```python
from build123d import *

# Parameters (mm, degrees)
SKETCH2_R           = 19.05
BOSS_EXTRUDE1_DEPTH = 62.484
SKETCH3_R           = 34.671
BOSS_EXTRUDE2_DEPTH = 12.7
SKETCH4_R           = 15.621
BOSS_EXTRUDE3_DEPTH = 19.05
SKETCH5_R           = 16.891
BOSS_EXTRUDE4_DEPTH = 2.54


with BuildPart() as part:
    # Sketch1 → Revolve1 (revolve)
    with BuildSketch(Plane.XY, mode=Mode.PRIVATE) as revolve1_sk:
        Polygon((0, 0), (0, 6.985), (16.761748485, 16.6624), (188.722, 16.6624), (188.722, 34.671), (201.422, 34.671), (201.422, 19.05), (300.99, 19.05), (300.99, 34.671), (326.39, 34.671), (332.329202219, 38.1), (484.729202219, 38.1), (484.729202219, 0), align=None)
    revolve(revolve1_sk.sketch.rotate(Axis((0, 0, 0), (1, 0, 0)), 90), axis=Axis((0, 0, 0), (1, 0, 0)))  # turned: the seam where the file's is

    # Sketch2 → Boss-Extrude1 (add)
    with BuildSketch(Plane(origin=(0, 0, 0), x_dir=(1, 0, 0), z_dir=(0, 1, 0))):
        with Locations(Location((251.206, 0, 0), (0, 0, 270))):  # turned: the seam where the file's is
            Circle(SKETCH2_R)
    extrude(amount=BOSS_EXTRUDE1_DEPTH)

    # Sketch3 → Boss-Extrude2 (add)
    with BuildSketch(Plane(origin=(0, 62.484, 0), x_dir=(1, 0, 0), z_dir=(0, 1, 0))):
        with Locations(Location((251.206, 0, 0), (0, 0, 270))):  # turned: the seam where the file's is
            Circle(SKETCH3_R)
    extrude(amount=-BOSS_EXTRUDE2_DEPTH)

    # Sketch4 → Boss-Extrude3 (add)
    with BuildSketch(Plane(origin=(484.729202219, 0, 0), x_dir=(0, 0, -1), z_dir=(1, 0, 0))):
        with Locations(Location((17.272, 0, 0), (0, 0, 180))):  # turned: the seam where the file's is
            Circle(SKETCH4_R)
    extrude(amount=BOSS_EXTRUDE3_DEPTH)

    # Sketch5 → Boss-Extrude4 (add)
    with BuildSketch(Plane(origin=(484.729202219, 0, 0), x_dir=(0, 0, -1), z_dir=(1, 0, 0))):
        with Locations(Location((-19.812, 0, 0), (0, 0, 180))):  # turned: the seam where the file's is
            Circle(SKETCH5_R)
    extrude(amount=BOSS_EXTRUDE4_DEPTH)


solid = part.part
```
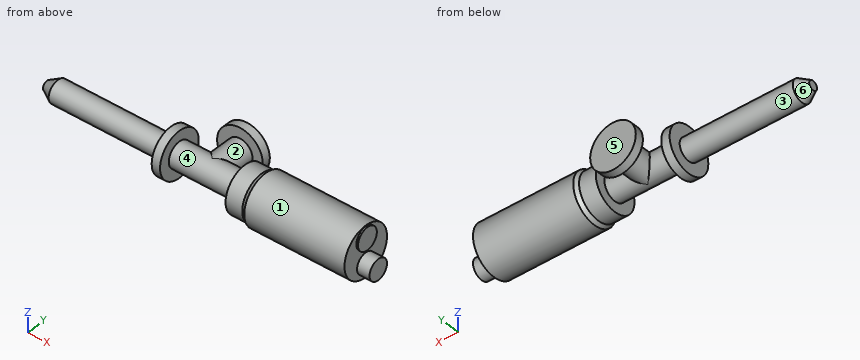
Geometry check sheet. Reference: the model listing, model coordinates, mm. Face numbers are marked on the shaded views. A direction names the side the tool comes from. Round coordinates to 2 decimals unless told otherwise and drop trailing zeros. Write each loop counter-clockwise with the first axis right and the second up, starting at its lowest first coordinate (ties: lowest second). Pieces come first, ordered by that corner, then holes. Notation, with made-up numbers: (-26.5, 25.5) -> (22.5, 25.5) arc R24 ccw to (22.5, 50.5) -> close; hole circle Ø1 at (-31.75, 63). An arc over 180 degrees is marked (long way). Put each result on its own line as item: value.
1) Cross-section at A-A, the plane x = 318. Enter the section's corners in (y, z), plus the area to 3 significant figures.
Recorded:
outline: circle Ø69.34 at (0, 0)
area: 3,780 mm2
2) Cross-section at C-C, the plane x = 78. Enter the section's corners in (y, z), plus the area to 3 significant figures.
Recorded:
outline: circle Ø33.32 at (0, 0)
area: 872 mm2
3) Release check for a two-part mould opening along X. For the marked faces 4, 5 and 6 record: pulls with the +X half, pulls with the -X half, needs draft (parallel to the pull), parting line crosses it, or undercut.
Recorded:
face 4: undercut
face 5: needs draft
face 6: pulls with the -X half
4) Depth check by flat-ended pin: P1, Ø10, axis at x = 233.5, y = 5, coming from the +Z side; P2, Ø1.5, axis at y = 19, z = 11.5, coming from the -X side; P3, Ø10, axis at y = 8.5, z = 4.5, coming from the +X side. Enter the tip coordinate at first touch or a pass-through.
Recorded:
P1: stops at z = 19.05
P2: stops at x = 188.72
P3: stops at x = 487.27
5) Thickness scan on probe 1 along X at (y, z) = (-30, 4); probe 2 along X at (y, z) = (-10.5, 16.5); probe 3 along Y at (x, z) = (224, 17). Record the ranges inside material, lowest first. Write a range as from..to.
Recorded:
probe 1: x = 188.72..201.42, 300.99..484.73
probe 2: x = 188.72..201.42, 300.99..487.27
probe 3: y = -8.6..8.6, 49.78..62.48
6) Access from +Z, -Z, +X, -X, +Y, -Y to the whole of each face (thin tool, end or side, straight path). Record for the marked faces 1, 2 and 3.
Recorded:
face 1: +X
face 2: none
face 3: -X
7) Cross-section at B-B, the plane z = 30.5. Give the number of separate pieces and of enclosed holes in the cut face, plus the area to 3 significant figures.
Recorded:
separate pieces: 3
enclosed holes: 0
area: 8,940 mm2
